Verification items for this drawing (mm, ordinates from the low corner). Give positions to 0.01 mm unless a question says otherwise; leave off trailing zeros. Loops run counter-clockwise (first coordinate to the right, second up) from the corner with the lowest first, then second, coordinate; pieces in that order, holes last. Notation, with made-up numbers: (83.5, -3.75) -> (99.5, -3.75) arc R20 cw to (99.5, 31.25) -> close; hole circle Ø10 at (-5.75, -16). An arc over 180 degrees is marked (long way). Answer as CSV lines item,"result". Start each with the question number.
(1) Gauge pin test, flat ends, axial feed: pin 1 Ø10 at (x, z) = (59, 9) entering from -Y; pin 2 Ø3 at (x, z) = (36, 26.5) entering from -Y; pin 3 Ø12 at (x, z) = (60, 19.5) entering from +Y. Record the tip position at first contact, or that the pin passes through.
(2) Material ranges on line 1 (Z direction, x = 80.5, y = 20); line 2 (X direction, y = 44.5, z = 9.5); line 3 (Y direction, x = 45, z = 12), recorded low to high. Write a range as from..to.
(3) Section check D-D on x = 61.5. Enter the section's corners in (y, z) (1 decimal).
(4) Section check C-C on z = 26.75. Enter the section's corners in (x, y), plus the area to 3 significant figures.
(5) Section check A-A on y = 45. Enter the section's corners in (x, z).
(6) Release check for a two-part mould opening along X. For the marked faces 1, 2 and 3 record: pulls with the +X half, pulls with the -X half, needs draft (parallel to the pull), parting line crosses it, or undercut.
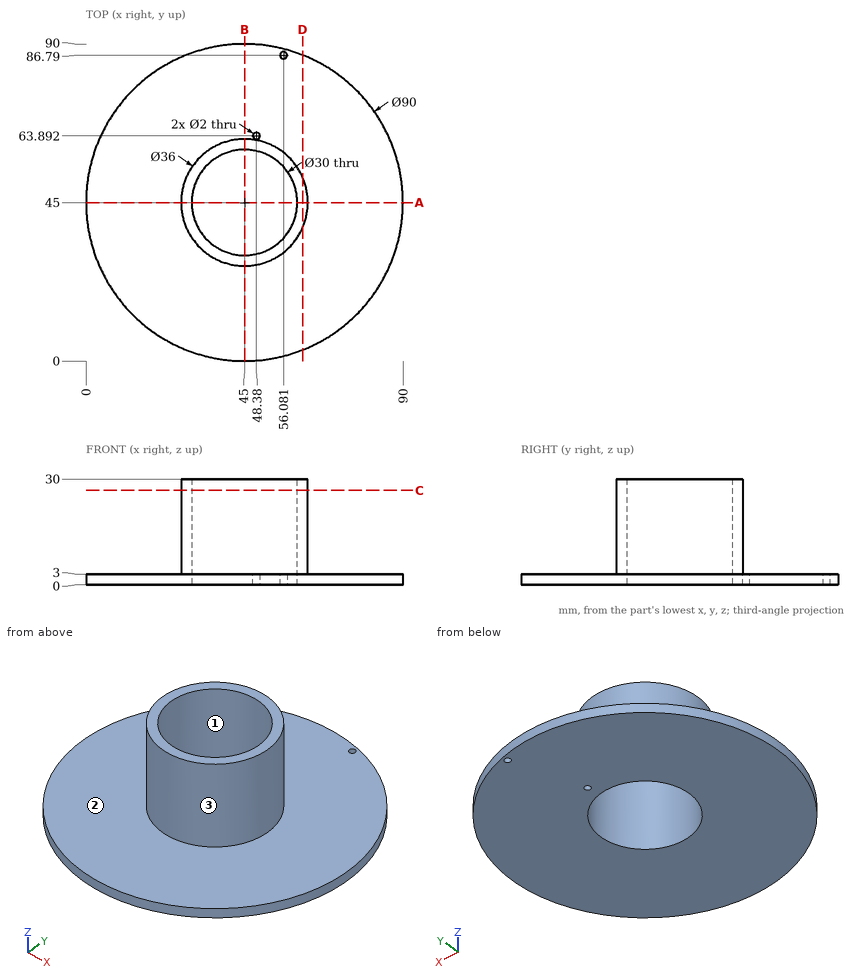
Working result:
1,pin 1,"stops at y = 29.41"
1,pin 2,"stops at y = 28.64"
1,pin 3,"stops at y = 60.59"
2,line 1,"z = 0..3"
2,line 2,"x = 27.01..30.01, 59.99..62.99"
2,line 3,"y = 27..30, 60..63"
3,outline,"(3.1, 0) -> (86.9, 0) -> (86.9, 3) -> (52.2, 3) -> (52.2, 30) -> (37.8, 30) -> (37.8, 3) -> (3.1, 3) -> close"
4,outline,"circle Ø36 at (45, 45); hole circle Ø30 at (45, 45)"
4,area,"311 mm^2"
5,outline,"(0, 0) -> (30, 0) -> (30, 30) -> (27, 30) -> (27, 3) -> (0, 3) -> close; (60, 0) -> (90, 0) -> (90, 3) -> (63, 3) -> (63, 30) -> (60, 30) -> close"
6,face 1,"undercut"
6,face 2,"needs draft"
6,face 3,"parting line crosses it"
